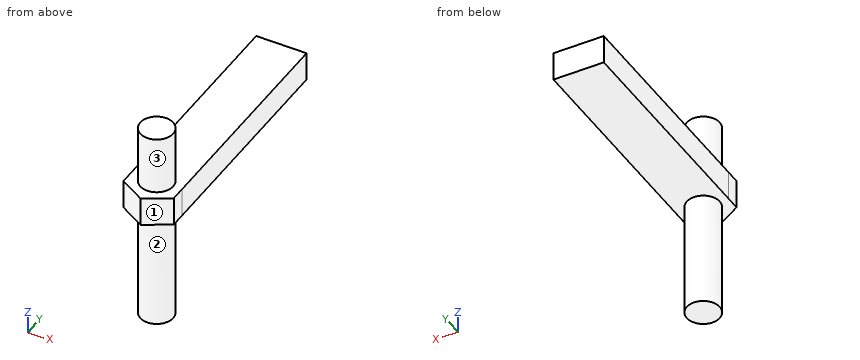
from build123d import *

# Parameters (mm, degrees)
CYLINDER025_R             = 1.7
CYLINDER025_DEPTH         = 21
BOX006_W                  = 23
BOX006_H                  = 5.2
BOX006_DEPTH              = 3
PRISM002_DEPTH            = 3
FUSION008_ROLL_ANGLE      = 180
FUSION008_PLACEMENT_ANGLE = 90


with BuildPart() as cilindro025:
    # Cylinder025 → Cylinder025 (new body)
    with BuildSketch(Plane.XY.offset(-6)):
        Circle(CYLINDER025_R)
    extrude(amount=CYLINDER025_DEPTH)


with BuildPart() as cubo005:
    # Box006 → Box006 (new body)
    with BuildSketch(Plane(origin=(0, -2.6, 0), x_dir=(1, 0, 0), z_dir=(0, 0, 1))):
        with Locations((11.5, 2.6)):
            Rectangle(BOX006_W, BOX006_H)
    extrude(amount=BOX006_DEPTH)


with BuildPart() as hueco_tornillo002:
    # Prism002 → Prism002 (new body)
    with BuildSketch(Plane.XY):
        Polygon((3, 0), (1.5, 2.598076), (-1.5, 2.598076), (-3, 0), (-1.5, -2.598076), (1.5, -2.598076), align=None)
    extrude(amount=PRISM002_DEPTH)

    # Fusion008: union Cilindro025, Cubo005
    add(cilindro025.part)
    add(cubo005.part)


with BuildPart() as hueco_tornillo002_1:
    # Fusion008 roll: moved
    add(hueco_tornillo002.part.rotate(Axis((0, 0, 0), (1, 0, 0)), FUSION008_ROLL_ANGLE))


with BuildPart() as hueco_tornillo002_2:
    # Fusion008 placement: moved
    add(hueco_tornillo002_1.part.moved(Location((159, 0, 62))).rotate(Axis((159, 0, 62), (0, 0, 1)), FUSION008_PLACEMENT_ANGLE))


solid = hueco_tornillo002_2.part
Source: CAD feature listing. Evaluate the final solid. Frame: model axes, mm. Face numbers are marked on the shaded views. A direction names the side the tool comes from. Coordinates: 2 decimals unless noted, no trailing zeros. Order: outer loops, then holes, each group sorted by start corner. A loop starts at its lowest first (then second) coordinate and runs counter-clockwise, first axis right, second up.
Item 1: Cut plane B-B (x = 157.7). Return loops of the section in (y, z), plus the area to 3 significant figures.
Output values:
outline: (-2.25, 59) - (-1.1, 59) - (-1.1, 47) - (1.1, 47) - (1.1, 59) - (23, 59) - (23, 62) - (1.1, 62) - (1.1, 68) - (-1.1, 68) - (-1.1, 62) - (-2.25, 62) - close
area: 115 mm2
Item 2: Cut plane C-C (y = 3.5). Return loops of the section in (x, z), plus the area to 3 significant figures.
Output values:
outline: (156.4, 59) - (161.6, 59) - (161.6, 62) - (156.4, 62) - close
area: 15.6 mm2
Item 3: Material intervals for line 1 (Z direction, x = 161.15, y = 2); line 2 (Y direction, x = 159, z = 49); line 3 (X direction, y = 0.5, z = 56.25), sorted ascending.
Output values:
line 1: z = 59 to 62
line 2: y = -1.7 to 1.7
line 3: x = 157.38 to 160.62
Item 4: First-contact query: P1, Ø3, axis at y = 1, z = 56.5, coming from the +X side; P2, Ø1, axis at x = 161, y = 14, coming from the -Z side. Flat tips, straight axial feed; report the tip coordinate or a pass-through.
Output values:
P1: stops at x = 160.7
P2: stops at z = 59
Item 5: Set-up query: the marked faces 1, 2 and 3. Return all of +Z, -Z, +X, -X, +Y, -Y with unobstructed straight access to the full face (end or side cutting, diameter ignored); none if empty.
Output values:
face 1: +Z, -Z, +X, -Y
face 2: -Z
face 3: +Z
Item 6: Cut plane D-D (z = 52.75). Return loops of the section in (x, y), plus the area to 3 significant figures.
Output values:
outline: circle Ø3.4 at (159, 0)
area: 9.08 mm2
